The listing builds one solid part. Answer for the finished solid, in the listing's coordinates (mm). Give positions to 0.01 mm unless a question says otherwise; leave off trailing zeros. Write each question's results on one line, items separated by ' | '. Start each with the question number.
Q1. Section A-A (z = 0.4) is taken. State how many separate pieces and enclosed holes the cut face has, plus the area to 3 significant figures.
Q2. A flat-ended cylindrical pin translates along its axis: pin 1 Ø1.5 at (x, y) = (84.5, -19.5) entering from -Z. Find the tip coordinate at first contact, or state that the pin passes through.
Q3. Find the intervals of material crossed by probe 1 along X at (y, z) = (35, 1.8); probe 2 along X at (y, z) = (34, 1.65), in increasing order.
```python
from build123d import *

# Parameters (mm, degrees)
F1_DEPTH = 2


with BuildPart() as f1:
    # F0 (on Top) → F1 (new body)
    with BuildSketch(Plane.XY):
        with BuildLine():
            ThreePointArc((275, 40), (273.535534, 43.535534), (270, 45))
            Line((270, 45), (-270, 45))
            ThreePointArc((-270, 45), (-273.535534, 43.535534), (-275, 40))
            Line((-275, 40), (-275, -40))
            ThreePointArc((-275, -40), (-273.535534, -43.535534), (-270, -45))
            Line((-270, -45), (270, -45))
            ThreePointArc((270, -45), (273.535534, -43.535534), (275, -40))
            Line((275, -40), (275, 40))
        make_face()
        with BuildLine():
            ThreePointArc((-251.5, -35), (-252.525126, -37.474874), (-255, -38.5))
            Line((-255, -38.5), (-265, -38.5))
            ThreePointArc((-265, -38.5), (-268.5, -35), (-265, -31.5))
            Line((-265, -31.5), (-255, -31.5))
            ThreePointArc((-255, -31.5), (-252.525126, -32.525126), (-251.5, -35))
        make_face(mode=Mode.SUBTRACT)
        with BuildLine():
            ThreePointArc((-121.5, -35), (-122.525126, -37.474874), (-125, -38.5))
            Line((-125, -38.5), (-135, -38.5))
            ThreePointArc((-135, -38.5), (-138.5, -35), (-135, -31.5))
            Line((-135, -31.5), (-125, -31.5))
            ThreePointArc((-125, -31.5), (-122.525126, -32.525126), (-121.5, -35))
        make_face(mode=Mode.SUBTRACT)
        with BuildLine():
            ThreePointArc((125, -38.5), (121.5, -35), (125, -31.5))
            Line((125, -31.5), (135, -31.5))
            ThreePointArc((135, -31.5), (137.474874, -32.525126), (138.5, -35))
            ThreePointArc((138.5, -35), (137.474874, -37.474874), (135, -38.5))
            Line((135, -38.5), (125, -38.5))
        make_face(mode=Mode.SUBTRACT)
        with BuildLine():
            ThreePointArc((255, -38.5), (251.5, -35), (255, -31.5))
            Line((255, -31.5), (265, -31.5))
            ThreePointArc((265, -31.5), (267.474874, -32.525126), (268.5, -35))
            ThreePointArc((268.5, -35), (267.474874, -37.474874), (265, -38.5))
            Line((265, -38.5), (255, -38.5))
        make_face(mode=Mode.SUBTRACT)
        with BuildLine():
            ThreePointArc((-265, 31.5), (-268.5, 35), (-265, 38.5))
            Line((-265, 38.5), (-255, 38.5))
            ThreePointArc((-255, 38.5), (-252.525126, 37.474874), (-251.5, 35))
            ThreePointArc((-251.5, 35), (-252.525126, 32.525126), (-255, 31.5))
            Line((-255, 31.5), (-265, 31.5))
        make_face(mode=Mode.SUBTRACT)
        with BuildLine():
            ThreePointArc((-135, 31.5), (-138.5, 35), (-135, 38.5))
            Line((-135, 38.5), (-125, 38.5))
            ThreePointArc((-125, 38.5), (-122.525126, 37.474874), (-121.5, 35))
            ThreePointArc((-121.5, 35), (-122.525126, 32.525126), (-125, 31.5))
            Line((-125, 31.5), (-135, 31.5))
        make_face(mode=Mode.SUBTRACT)
        with BuildLine():
            ThreePointArc((125, 31.5), (121.5, 35), (125, 38.5))
            Line((125, 38.5), (135, 38.5))
            ThreePointArc((135, 38.5), (137.474874, 37.474874), (138.5, 35))
            ThreePointArc((138.5, 35), (137.474874, 32.525126), (135, 31.5))
            Line((135, 31.5), (125, 31.5))
        make_face(mode=Mode.SUBTRACT)
        with BuildLine():
            ThreePointArc((255, 31.5), (251.5, 35), (255, 38.5))
            Line((255, 38.5), (265, 38.5))
            ThreePointArc((265, 38.5), (267.474874, 37.474874), (268.5, 35))
            ThreePointArc((268.5, 35), (267.474874, 32.525126), (265, 31.5))
            Line((265, 31.5), (255, 31.5))
        make_face(mode=Mode.SUBTRACT)
    extrude(amount=F1_DEPTH)


solid = f1.part
```
Answers below:
1) separate pieces: 1 | enclosed holes: 8 | area: 48,600 mm2
2) pin 1: stops at z = 0
3) probe 1: x = -275 to -268.5, -251.5 to -138.5, -121.5 to 121.5, 138.5 to 251.5, 268.5 to 275 | probe 2: x = -275 to -268.35, -251.65 to -138.35, -121.65 to 121.65, 138.35 to 251.65, 268.35 to 275
